Verification items for the finished model (mm, model axes). A direction names the side the tool comes from. Give positions to 0.01 mm unless a question says otherwise; leave off trailing zeros. Write each loop counter-clockwise with the first axis right and the second up, starting at its lowest first coordinate (ties: lowest second). Pieces come first, ordered by that corner, then holes. Notation, with made-up numbers: (65, 48.25) -> (100, 48.25) arc R23 cw to (100, 65.25) -> close; hole circle Ø8 at (-29.75, 79.25). An arc over 180 degrees is marked (long way). Write item = value, one per line.
from build123d import *

# Parameters (mm, degrees)
F0_R     = 29.871853
F1_DEPTH = 15
F2_R     = 24.016909
F3_DEPTH = 6
F4_R     = 3
F5_DEPTH = 25


with BuildPart() as f1:
    # F0 (on Front) → F1 (new body)
    with BuildSketch(Plane.XZ):
        Circle(F0_R)
    extrude(amount=F1_DEPTH)

    # F2 (on face) → F3 (cut)
    with BuildSketch(Plane(origin=(0, 0, 0), x_dir=(-1, 0, 0), z_dir=(0, 1, 0))):
        Circle(F2_R)
    extrude(amount=-F3_DEPTH, mode=Mode.SUBTRACT)

    # F4 (on face) → F5 (cut)
    with BuildSketch(Plane(origin=(0, -6, 0), x_dir=(-1, 0, 0), z_dir=(0, 1, 0))):
        with Locations((0, 11.006043)):
            Circle(F4_R)
        with Locations((0, -9.993957)):
            Circle(F4_R)
    extrude(amount=-F5_DEPTH, mode=Mode.SUBTRACT)


solid = f1.part
Item 1: Go/stop test with flat-tipped pins: P1, Ø2, axis at x = -11, y = -4, coming from the +Z side; P2, Ø6, axis at y = -6.5, z = 7, coming from the +X side; P3, Ø1, axis at x = -22, y = -7, coming from the -Z side; P4, Ø5.5, axis at x = 0, z = 11.01, coming from the -Y side. Record where each tip stops, or that it passes through.
Response values:
P1 = 28.15
P2 = 29.6
P3 = -20.74
P4 = through
Item 2: Sectioned sample at C-C on y = -2.5. Record the cut outline in (x, z).
Response values:
outline = circle Ø59.74 at (0, 0); hole circle Ø48.03 at (0, 0)
Item 3: Sectioned sample at B-B on z = 0. Record the cut outline in (x, y), then the cut area to 3 significant figures.
Response values:
outline = (-29.87, -15) -> (29.87, -15) -> (29.87, 0) -> (24.02, 0) -> (24.02, -6) -> (-24.02, -6) -> (-24.02, 0) -> (-29.87, 0) -> close
area = 608 mm^2
Item 4: Mould release check, pull along Z, two halves, no side actions. Record for faces 1 (the flat face through (0, -15, 0)), 2 (the cylindrical face through (-22.017, -7.395, 20.189)), 3 (the cylindrical face through (5.206, -2.958, -23.446)): +Z half, -Z half, draft (parallel to the pull), parting line (faces both ways), or undercut.
Response values:
face_1 = draft
face_2 = parting line
face_3 = undercut
Item 5: Sectioned sample at A-A on x = 0. Record the cut outline in (y, z), then the cut area to 3 significant figures.
Response values:
outline = (-15, -29.87) -> (0, -29.87) -> (0, -24.02) -> (-6, -24.02) -> (-6, -12.99) -> (-15, -12.99) -> close; (-15, -6.99) -> (-6, -6.99) -> (-6, 8.01) -> (-15, 8.01) -> close; (-15, 14.01) -> (-6, 14.01) -> (-6, 24.02) -> (0, 24.02) -> (0, 29.87) -> (-15, 29.87) -> close
area = 500 mm^2
Item 6: Sectioned sample at D-D on x = 16. Record the cut outline in (y, z), then the cut area to 3 significant figures.
Response values:
outline = (-15, -25.23) -> (0, -25.23) -> (0, -17.91) -> (-6, -17.91) -> (-6, 17.91) -> (0, 17.91) -> (0, 25.23) -> (-15, 25.23) -> close
area = 542 mm^2
Item 7: Material ranges on line 1 (Z direction, x = 0, y = -7.75); line 2 (Z direction, x = -12, y = -3.25); line 3 (Y direction, x = -10.5, z = 3), recorded low to high.
Response values:
line_1 = -29.87 to -12.99, -6.99 to 8.01, 14.01 to 29.87
line_2 = -27.36 to -20.8, 20.8 to 27.36
line_3 = -15 to -6
Item 8: Set-up check for faces 4 (the flat face through (0, -6, 0)), 5 (the flat face through (2.1, 0, 24.5)): record each of +Z, -Z, +X, -X, +Y, -Y from which the full face is reachable in a straight line by a thin tool's end or side.
Response values:
face_4 = +Y
face_5 = +Z, -Z, +X, -X, +Y
